Part model, mm, in its own coordinate system. A direction names the side the tool comes from. Round coordinates to 2 decimals unless told otherwise and drop trailing zeros. Order: outer loops, then holes, each group sorted by start corner. A loop starts at its lowest first (then second) coordinate and runs counter-clockwise, first axis right, second up. Notation, with made-up numbers: (12.5, -30) - (50.5, -30) arc R19 cw to (50.5, -7) - close; hole circle Ø2 at (-34, -17.5). An arc over 180 degrees is marked (long way). Return JSON: item names as keys, results as strings. Group by question number.
Item 1: Saw through at B-B on z = 1.5. List the corners of the cut face in (x, y), and give its area (3 significant figures).
Item 2: Probe probe 1 along Y at (x, z) = (0, 6.5); probe 2 along Y at (x, z) = (0, 15); probe 3 along Z at (x, y) = (3, 2.75). List the from-to ranges inside material, lowest first.
Item 3: Tool access for faces 4 (the face through (2.931, 0.923, 12.629)), 5 (the face through (-3.546, -2.086, 1.628)), 6 (the face through (4, 2, 0)): list every direction of +Z, -Z, +X, -X, +Y, -Y with a clear straight run to the whole face (end or side of a thin tool).
Item 4: Saw through at D-D on x = -3.5. List the corners of the cut face in (y, z).
Item 5: Saw through at A-A on x = 0. List the corners of the cut face in (y, z).
Item 6: Drop flat-ended pins along their axis: pin 1 (2 mm diameter, centred on x = 5, z = 2, fed in from +Y); pin 2 (4 mm diameter, centred on x = 1.5, y = -1, fed in from -Z); pin 3 (2 mm diameter, centred on x = 5, y = -0.5, fed in from +Z). Give the stop position or say it passes through.
Item 7: Saw through at C-C on y = -2.5. List the corners of the cut face in (x, z).
Item 8: Two-plate mould, pull along Y, no slides. Class faces 1 (the face through (3, 2, 7.62)), 2 (the face through (-1.38, -6.2, 3.76)), 3 (the face through (3.546, 2.086, 1.628)): released by +Y, released by -Y, zero draft, split by the parting line, or undercut.
```python
from build123d import *

# Parameters (mm, degrees)
F0_R     = 6.35
F1_DEPTH = 7.62
F2_R     = 3.0734
F3_DEPTH = 10.16
F4_R     = 2.2225
F5_DEPTH = 17.781
F7_DEPTH = 3.302


with BuildPart() as f1:
    # F0 (on Top) → F1 (new body)
    with BuildSketch(Plane.XY):
        Circle(F0_R)
    extrude(amount=F1_DEPTH)

    # F2 (on face) → F3 (join)
    with BuildSketch(Plane.XY.offset(7.62)):
        Circle(F2_R)
    extrude(amount=F3_DEPTH)

    # F4 (on face) → F5 (cut, through all)
    with BuildSketch(Plane.XY.offset(17.78)):
        Circle(F4_R)
    extrude(amount=-F5_DEPTH, mode=Mode.SUBTRACT)

    # F6 (on face) → F7 (cut)
    with BuildSketch(Plane(origin=(0, 0, 0), x_dir=(1, 0, 0), z_dir=(0, 0, -1))):
        Polygon((2.3749, 4.113447), (-2.3749, 4.113447), (-4.7498, 0), (-2.3749, -4.113447), (2.3749, -4.113447), (4.7498, 0), align=None)
    extrude(amount=-F7_DEPTH, mode=Mode.SUBTRACT)


solid = f1.part
```
Filled in:
{
 "1": {"outline": "circle Ø12.7 at (0, 0); hole (-4.75, 0) - (-2.37, -4.11) - (2.37, -4.11) - (4.75, 0) - (2.37, 4.11) - (-2.37, 4.11) - close", "area": "68.1 mm^2"},
 "2": {"probe 1": "y = -6.35 to -2.22, 2.22 to 6.35", "probe 2": "y = -3.07 to -2.22, 2.22 to 3.07", "probe 3": "z = 3.3 to 7.62"},
 "3": {"face 4": "+Z", "face 5": "-Z", "face 6": "-Z, +X, -X, +Y, -Y"},
 "4": {"outline": "(-5.3, 0) - (-2.16, 0) - (-2.16, 3.3) - (2.16, 3.3) - (2.16, 0) - (5.3, 0) - (5.3, 7.62) - (-5.3, 7.62) - close"},
 "5": {"outline": "(-6.35, 0) - (-4.11, 0) - (-4.11, 3.3) - (-2.22, 3.3) - (-2.22, 17.78) - (-3.07, 17.78) - (-3.07, 7.62) - (-6.35, 7.62) - close; (2.22, 3.3) - (4.11, 3.3) - (4.11, 0) - (6.35, 0) - (6.35, 7.62) - (3.07, 7.62) - (3.07, 17.78) - (2.22, 17.78) - close"},
 "6": {"pin 1": "stops at y = 4.93", "pin 2": "stops at z = 3.3", "pin 3": "stops at z = 7.62"},
 "7": {"outline": "(-5.84, 0) - (-3.31, 0) - (-3.31, 3.3) - (3.31, 3.3) - (3.31, 0) - (5.84, 0) - (5.84, 7.62) - (1.79, 7.62) - (1.79, 17.78) - (-1.79, 17.78) - (-1.79, 7.62) - (-5.84, 7.62) - close"},
 "8": {"face 1": "zero draft", "face 2": "split by the parting line", "face 3": "undercut"}
}
